Geometry check sheet. Reference: the model listing, model coordinates, mm. Give positions to 0.01 mm unless a question says otherwise; leave off trailing zeros.
(1) Cross-section at A-A (z = 266.5). Count the separate pieces of the cut face and the enclosed holes in it, and give its area (3 significant figures).
(2) Depth check by flat-ended pin: P1, Ø4, axis at x = -22.5, z = 798, coming from the -Y side; P2, Ø3, axis at x = -8.5, y = 8, coming from the -Z side. Enter the tip coordinate at first touch or a pass-through.
(3) Thickness scan on line 1 along Y through (x, z) = (20.5, 328); line 2 along X through (y, z) = (8, 146); line 3 along X through (y, z) = (-12.5, 492.5). Record the ranges inside material, lowest first.
```python
from build123d import *

# Parameters (mm, degrees)
SKETCH_1_R      = 2.5
SKETCH_1_R_2    = 3.4
EXTRUDE_1_DEPTH = 1000


with BuildPart() as part:
    # 草图1 → 凸台-拉伸1 (new body)
    with BuildSketch(Plane.XY):
        with BuildLine():
            Line((-17.204286219, -18.118225585), (6.295713781, -18.118225585))
            Line((6.295713781, -18.118225585), (6.295713781, -15.818225585))
            Line((6.295713781, -15.818225585), (4.345713781, -15.818225585))
            Line((4.345713781, -15.818225585), (4.345713781, -10.018225585))
            ThreePointArc((4.345713781, -10.018225585), (9.545713781, -7.418225585), (14.745713781, -10.018225585))
            Line((14.745713781, -10.018225585), (14.745713781, -15.818225585))
            Line((14.745713781, -15.818225585), (12.795713781, -15.818225585))
            Line((12.795713781, -15.818225585), (12.795713781, -18.118225585))
            Line((12.795713781, -18.118225585), (23.545713781, -18.118225585))
            ThreePointArc((23.545713781, -18.118225585), (24.252820562, -17.825332366), (24.545713781, -17.118225585))
            Line((24.545713781, -17.118225585), (24.545713781, -6.368225585))
            Line((24.545713781, -6.368225585), (22.245713781, -6.368225585))
            Line((22.245713781, -6.368225585), (22.245713781, -8.318225585))
            Line((22.245713781, -8.318225585), (16.445713781, -8.318225585))
            ThreePointArc((16.445713781, -8.318225585), (13.845713781, -3.118225585), (16.445713781, 2.081774415))
            Line((16.445713781, 2.081774415), (22.245713781, 2.081774415))
            Line((22.245713781, 2.081774415), (22.245713781, 0.131774415))
            Line((22.245713781, 0.131774415), (24.545713781, 0.131774415))
            Line((24.545713781, 0.131774415), (24.545713781, 10.881774415))
            ThreePointArc((24.545713781, 10.881774415), (24.252820562, 11.588881197), (23.545713781, 11.881774415))
            Line((23.545713781, 11.881774415), (12.795713781, 11.881774415))
            Line((12.795713781, 11.881774415), (12.795713781, 9.581774415))
            Line((12.795713781, 9.581774415), (14.745713781, 9.581774415))
            Line((14.745713781, 9.581774415), (14.745713781, 3.781774415))
            ThreePointArc((14.745713781, 3.781774415), (9.545713781, 1.181774415), (4.345713781, 3.781774415))
            Line((4.345713781, 3.781774415), (4.345713781, 9.581774415))
            Line((4.345713781, 9.581774415), (6.295713781, 9.581774415))
            Line((6.295713781, 9.581774415), (6.295713781, 11.881774415))
            Line((6.295713781, 11.881774415), (-17.204286219, 11.881774415))
            Line((-17.204286219, 11.881774415), (-17.204286219, 9.581774415))
            Line((-17.204286219, 9.581774415), (-15.254286219, 9.581774415))
            Line((-15.254286219, 9.581774415), (-15.254286219, 3.781774415))
            ThreePointArc((-15.254286219, 3.781774415), (-20.454286219, 1.181774415), (-25.654286219, 3.781774415))
            Line((-25.654286219, 3.781774415), (-25.654286219, 9.581774415))
            Line((-25.654286219, 9.581774415), (-23.704286219, 9.581774415))
            Line((-23.704286219, 9.581774415), (-23.704286219, 11.881774415))
            Line((-23.704286219, 11.881774415), (-34.454286219, 11.881774415))
            ThreePointArc((-34.454286219, 11.881774415), (-35.161393, 11.588881197), (-35.454286219, 10.881774415))
            Line((-35.454286219, 10.881774415), (-35.454286219, 0.131774415))
            Line((-35.454286219, 0.131774415), (-33.154286219, 0.131774415))
            Line((-33.154286219, 0.131774415), (-33.154286219, 2.081774415))
            Line((-33.154286219, 2.081774415), (-27.354286219, 2.081774415))
            ThreePointArc((-27.354286219, 2.081774415), (-24.754286219, -3.118225585), (-27.354286219, -8.318225585))
            Line((-27.354286219, -8.318225585), (-33.154286219, -8.318225585))
            Line((-33.154286219, -8.318225585), (-33.154286219, -6.368225585))
            Line((-33.154286219, -6.368225585), (-35.454286219, -6.368225585))
            Line((-35.454286219, -6.368225585), (-35.454286219, -17.118225585))
            ThreePointArc((-35.454286219, -17.118225585), (-35.161393, -17.825332366), (-34.454286219, -18.118225585))
            Line((-34.454286219, -18.118225585), (-23.704286219, -18.118225585))
            Line((-23.704286219, -18.118225585), (-23.704286219, -15.818225585))
            Line((-23.704286219, -15.818225585), (-25.654286219, -15.818225585))
            Line((-25.654286219, -15.818225585), (-25.654286219, -10.018225585))
            ThreePointArc((-25.654286219, -10.018225585), (-20.454286219, -7.418225585), (-15.254286219, -10.018225585))
            Line((-15.254286219, -10.018225585), (-15.254286219, -15.818225585))
            Line((-15.254286219, -15.818225585), (-17.204286219, -15.818225585))
            Line((-17.204286219, -15.818225585), (-17.204286219, -18.118225585))
        make_face()
        with Locations((-20.454286219, -3.118225585)):
            Circle(SKETCH_1_R, mode=Mode.SUBTRACT)
        with Locations((-30.554286219, -13.218225585)):
            Circle(SKETCH_1_R_2, mode=Mode.SUBTRACT)
        with Locations((-30.554286219, 6.981774415)):
            Circle(SKETCH_1_R_2, mode=Mode.SUBTRACT)
        with Locations((19.645713781, -13.218225585)):
            Circle(SKETCH_1_R_2, mode=Mode.SUBTRACT)
        with Locations((19.645713781, 6.981774415)):
            Circle(SKETCH_1_R_2, mode=Mode.SUBTRACT)
        with Locations((9.545713781, -3.118225585)):
            Circle(SKETCH_1_R, mode=Mode.SUBTRACT)
        with BuildLine():
            Line((2.045713781, -15.818225585), (2.045713781, -8.718225585))
            ThreePointArc((2.045713781, -8.718225585), (5.245713781, -3.118225585), (2.045713781, 2.481774415))
            Line((2.045713781, 2.481774415), (2.045713781, 9.581774415))
            Line((2.045713781, 9.581774415), (-12.954286219, 9.581774415))
            Line((-12.954286219, 9.581774415), (-12.954286219, 2.481774415))
            ThreePointArc((-12.954286219, 2.481774415), (-16.154286219, -3.118225585), (-12.954286219, -8.718225585))
            Line((-12.954286219, -8.718225585), (-12.954286219, -15.818225585))
            Line((-12.954286219, -15.818225585), (2.045713781, -15.818225585))
        make_face(mode=Mode.SUBTRACT)
    extrude(amount=EXTRUDE_1_DEPTH)


solid = part.part
```
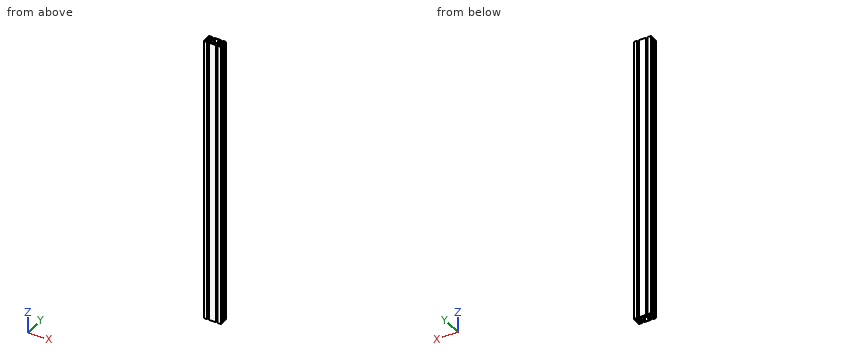
Reply:
1. separate pieces: 1
1. enclosed holes: 7
1. area: 618 mm2
2. P1: stops at y = -18.12
2. P2: passes through
3. line 1: y = -18.12 to -16.51, -9.93 to -8.32, 2.08 to 3.69, 10.27 to 11.88
3. line 2: x = -35.45 to -33.8, -27.31 to -25.65, -15.25 to -12.95, 2.05 to 4.35, 14.75 to 16.4, 22.89 to 24.55
3. line 3: x = -35.45 to -33.88, -27.23 to -25.65, -15.25 to -12.95, 2.05 to 4.35, 14.75 to 16.32, 22.97 to 24.55
